Autodesk Inventor part; units mm, degrees
ref_plane "Work Plane2" through (-8.159, -4.964, 0.6) normal (0, 0, -1) x (0, 1, 0)
ref_plane "YZ Plane" through (0, 0, 0) normal (1, 0, 0) x (0, 1, 0)
ref_plane "XZ Plane" through (0, 0, 0) normal (0, 1, 0) x (-1, 0, 0)
ref_plane "Work Plane1" through (-1, 1, 0) normal (0, 0, 1) x (1, 0, 0)
sketch "Sketch1" plane through (-1, 1, 0) normal (0, 0, 1) x (1, 0, 0)
  circle A0 centre (-8, 7.7) radius 1.35
  circle A1 centre (-8, -7.7) radius 1.35
  circle A2 centre (-1.159, 0.036) radius 6 construction
  line L0 (-12, 11.7) -> (6, 11.7)
  line L1 (6, 11.7) -> (6, -11.7)
  line L2 (6, -11.7) -> (-12, -11.7)
  line L3 (-12, -11.7) -> (-12, 11.7)
  point P0 (1, -1)
  dimension "d0" = 18
  dimension "d2" = 4
  dimension "d3" = 4
  dimension "d12" = 4
extrude "Extrusion1" add sketch "Sketch1" along normal blind 1
sketch "Sketch2" plane through (-1, 1, 1) normal (0, 0, 1) x (1, 0, 0)
  circle A0 centre (-1.159, 0.036) radius 6
  circle A1 centre (-1.159, 0.036) radius 5
  point P0 (1, -1)
  dimension "d6" = 10
extrude "Extrusion2" cut sketch "Sketch2" against normal through all contours A1
sketch "Sketch3" plane through (-1, 1, 0) normal (0, 0, -1) x (-1, 0, 0)
  circle A0 centre (1.159, 0.036) radius 5
  circle A1 centre (1.159, 0.036) radius 6.25
  point P0 (-1, -1)
  dimension "d9" = 12.5
ref_plane "Work Plane2" through (-8.159, -4.964, 0.6) normal (0, 0, -1) x (0, 1, 0)
extrude "Extrusion3" cut sketch "Sketch3" against normal up to surface (0.6 mm away)
sketch "Sketch4" plane through (-1, 1, 0) normal (0, 0, -1) x (-1, 0, 0)
  circle A0 centre (8, 7.7) radius 1.35
  circle A1 centre (8, -7.7) radius 1.35
  circle A2 centre (1.159, 0.036) radius 6.25
  line L0 (8, 9.05) -> (0.0063, 9.05)
  line L1 (0.0063, 9.05) -> (0.0063, 6.35)
  line L2 (0.0063, 6.35) -> (8, 6.35)
  line L3 (8, 6.35) -> (8, 9.05)
  line L4 (8, -6.35) -> (0.0063, -6.35)
  line L5 (0.0063, -6.35) -> (0.0063, -9.05)
  line L6 (0.0063, -9.05) -> (8, -9.05)
  line L7 (8, -9.05) -> (8, -6.35)
  line L8 (0.0063, -6.35) -> (0.0063, -6.1068)
  line L9 (3.5216, -6.35) -> (3.5216, -5.7502)
  circle A3 centre (1.159, 0.036) radius 6.25
  line L10 (3.9246, 6.35) -> (3.9246, 5.6409)
  line L11 (0.0063, 6.35) -> (0.0063, 6.1788)
  point P0 (-1, -1)
extrude "Extrusion4" cut sketch "Sketch4" against normal blind 0.5 contours L3 A0 | A0 L2 L1 L0 | L10 A2 L11 L2 | A2 | A2 L9 L4 L8 | L4 A1 L6 L5 | L7 A1 picked at (7.3128, 7.4828) picked at (7.2624, -7.8211)
sketch "Sketch5" plane through (-1, 1, 1) normal (0, 0, 1) x (1, 0, 0)
  circle A0 centre (-8, 7.7) radius 0.5
  circle A1 centre (-8, 7.7) radius 1.35
  circle A2 centre (-8, -7.7) radius 0.5
  circle A3 centre (-8, -7.7) radius 1.35
  arc A4 (-8, 9.05) -> (-8, 6.35) centre (-8, 7.7) ccw
  circle A5 centre (-8, 7.7) radius 2.5
  circle A6 centre (-8, -7.7) radius 2.5
  point P0 (1, -1)
  dimension "d15" = 5
  dimension "d16" = 5
extrude "Extrusion5" add sketch "Sketch5" along normal blind 2 contours A5 | A6
properties part number "00_PDMS_chamber_fluidic_v0"
Part model, mm, in its own coordinate system. A direction names the side the tool comes from. Coordinates: 2 decimals unless noted, no trailing zeros. Loops run counter-clockwise (first coordinate to the right, second up) from the corner with the lowest first, then second, coordinate; pieces in that order, holes last. Notation, with made-up numbers: (57, 55.5) -> (64, 55.5) arc R22 cw to (64, 69.5) -> close; hole circle Ø2 at (21.25, 28.25). An arc over 180 degrees is marked (long way). Use a Markdown table: item, result. Add a question column.
Item 1: Which spindle directions (+Z, -Z, +X, -X, +Y, -Y) get a long thin tool onto all of the face, cutting with end or side? Do faces 4 (the cylindrical face through (-9.33, 6.22, 1.99)), 5 (the flat face through (-4, 6, 0.6)), 6 (the flat face through (-3.9, -10.7, 0.5)). Say none if no direction does.
Item 2: Flat gauge pins, fed straight in: P1, Ø4, axis at x = -6, y = -0.5, coming from the -Z side; P2, Ø1.6, axis at x = -3, y = -7, coming from the -Z side; P3, Ø3, axis at x = -9, y = -4.5, coming from the -Z side. Where does each tip first touch, or does it go through?
Item 3: Pull direction X, two halves, no side cores. Call faces 1 (the cylindrical face through (-9.54, -4.26, 1.99)), 2 (the flat face through (-4, -7, 0.5)), 3 (the flat face through (-4.1, 12.7, 0.5)): +X half, -X half, draft (parallel to the pull), parting line (faces both ways), or undercut.
Item 4: Band-saw the part on B-B on z = 1.75. Write the cut outline in (x, y).
Item 5: Band-saw the part on C-C on x = 1.25. Write the cut outline in (y, z), plus the area to 3 significant figures.
Item 6: Band-saw the part on D-D on x = -8.75. Give the number of separate pieces and of enclosed holes in the cut face, plus the area to 3 significant figures.
Item 7: Probe probe 1 along Y at (x, z) = (-9, 2.8); probe 2 along X at (y, z) = (8.75, 1.95); probe 3 along Z at (x, y) = (-6.25, 7.75). List the from-to ranges inside material, lowest first.
Item 8: Band-saw the part on A-A on y = -6.7. Write the cut outline in (x, z).
Geometry says:
| question | item | result |
|---|---|---|
| 1 | face 4 | +Z |
| 1 | face 5 | -Z |
| 1 | face 6 | +Z, -Z, +X, -X, -Y |
| 2 | P1 | z = 0.6 |
| 2 | P2 | z = 0.5 |
| 2 | P3 | z = 0 |
| 3 | face 1 | parting line |
| 3 | face 2 | undercut |
| 3 | face 3 | draft |
| 4 | outline | circle Ø5 at (-9, -6.7); circle Ø5 at (-9, 8.7); hole circle Ø2.7 at (-9, -6.7); hole circle Ø2.7 at (-9, 8.7) |
| 5 | outline | (-10.7, 0) -> (-4.2, 0) -> (-4.2, 0.6) -> (-2.62, 0.6) -> (-2.62, 1) -> (-10.7, 1) -> close; (4.69, 0.6) -> (6.27, 0.6) -> (6.27, 0) -> (12.7, 0) -> (12.7, 1) -> (4.69, 1) -> close |
| 5 | area | 14.2 mm² |
| 6 | separate pieces | 3 |
| 6 | enclosed holes | 0 |
| 6 | area | 27.3 mm² |
| 7 | probe 1 | -9.2 to -8.05, -5.35 to -4.2, 6.2 to 7.35, 10.05 to 11.2 |
| 7 | probe 2 | -11.5 to -10.35, -7.65 to -6.5 |
| 7 | probe 3 | 0.5 to 1 |
| 8 | outline | (-13, 0) -> (-10.35, 0) -> (-10.35, 3) -> (-11.5, 3) -> (-11.5, 1) -> (-13, 1) -> close; (-7.65, 0.5) -> (-1.01, 0.5) -> (-1.01, 0) -> (5, 0) -> (5, 1) -> (-6.5, 1) -> (-6.5, 3) -> (-7.65, 3) -> close |
